Can you work these out from the model? Positions are in its coordinate system, mm. Face numbers are marked on the shaded views. A direction names the side the tool comes from. Give positions to 0.01 mm unless a question says otherwise; leave off trailing zeros. Order: outer loops, then holes, each group sorted by start corner. A loop starts at its lowest first (then second) coordinate and runs counter-clockwise, first axis right, second up. Notation, with made-up numbers: (-7.75, 86) - (46.25, 86) arc R15 ccw to (46.25, 96) - close; hole circle Ø7 at (75, -13.75). An arc over 180 degrees is marked (long way). Return JSON: item names as keys, results as strings.
```python
from build123d import *

# Parameters (mm, degrees)
BOSS_EXTRUDE1_DEPTH    = 66.04
F_10_CLEARANCE_HOLE1_D = 5.1054


with BuildPart() as part:
    # Sketch2 → Boss-Extrude1 (new body)
    with BuildSketch(Plane.XY):
        Polygon((0, 0), (114.3, 0), (114.3, -8.89), (104.775, -8.89), (104.775, -15.24), (9.525, -15.24), (9.525, -8.89), (0, -8.89), align=None)
    extrude(amount=BOSS_EXTRUDE1_DEPTH)

    # #10 Clearance Hole1 (through all)
    with Locations(Plane(origin=(4.826, 0, 12.7), x_dir=(0, 0, 1), z_dir=(0, 1, 0))):
        with Locations((0, 0), (38.1, 0), (38.1, 104.648), (0, 104.648)):
            Hole(F_10_CLEARANCE_HOLE1_D / 2)


solid = part.part
```
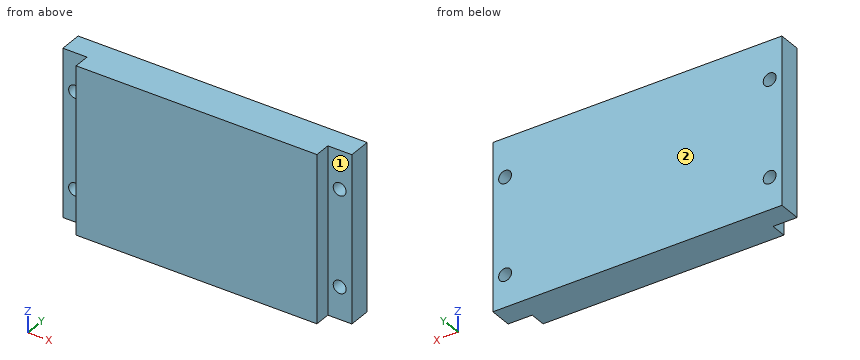
1. Suppose I cut it at A-A (z = 50.8). List the corners of the cut face in (x, y) for me (3 decimals), plus the area to 3 significant figures.
Checks:
{"outline": "(0, -8.89) - (2.273, -8.89) - (2.273, 0) - (0, 0) - close; (7.379, -8.89) - (9.525, -8.89) - (9.525, -15.24) - (104.775, -15.24) - (104.775, -8.89) - (106.921, -8.89) - (106.921, 0) - (7.379, 0) - close; (112.027, -8.89) - (114.3, -8.89) - (114.3, 0) - (112.027, 0) - close", "area": "1,530 mm^2"}
2. On a 3-axis mill with a long thin cutter (end or side, diameter ignored), from which of +Z, -Z, +X, -X, +Y, -Y can I reach the whole of each face in a straight line? I mean the marked faces 1 and 2. Say none if no direction works.
Checks:
{"face 1": "+Z, -Z, +X, -Y", "face 2": "+Z, -Z, +X, -X, +Y"}
3. For pin 1 Ø6.5 at (x, z) = (109.474, 50.8) entering from -Y; pin 2 Ø7 at (y, z) = (-13.5, 46) entering from -X (3 decimals); pin 3 Ø3 at (x, z) = (4.826, 50.8) entering from +Y; pin 4 Ø5 at (y, z) = (-13, 20.5) entering from +X (3 decimals), each with a flat end and sliding along its axis, tell me the tip position at first contact or that it passes through.
Checks:
{"pin 1": "y = -8.89", "pin 2": "x = 9.525", "pin 3": "through", "pin 4": "x = 104.775"}
4. Suppose I cut it at B-B (z = 39.5). List the corners of the cut face in (x, y) for me (3 decimals).
Checks:
{"outline": "(0, -8.89) - (9.525, -8.89) - (9.525, -15.24) - (104.775, -15.24) - (104.775, -8.89) - (114.3, -8.89) - (114.3, 0) - (0, 0) - close"}
5. If I drill on L1, parallel to X at y = -4, z = 12.7; L2, parallel to X at y = -7.5, z = 50; L3, parallel to X at y = -10.25, z = 41 (3 decimals), over which ranges is the centre line in solid material (lowest first)? Write a range as [from, to].
Checks:
{"L1": "[0, 2.27], [7.38, 106.92], [112.03, 114.3]", "L2": "[0, 2.4], [7.25, 107.05], [111.9, 114.3]", "L3": "[9.525, 104.775]"}
